from build123d import *

# Parameters (mm, degrees)
SKETCH_2_W      = 48
SKETCH_2_H      = 48
SKETCH_2_W_2    = 40
SKETCH_2_H_2    = 40
EXTRUDE_1_DEPTH = 100
SKETCH_3_W      = 48
SKETCH_3_H      = 48
SKETCH_3_W_2    = 40
SKETCH_3_H_2    = 40
EXTRUDE_2_DEPTH = 40
SKETCH_4_W      = 48
SKETCH_4_H      = 48
SKETCH_4_W_2    = 40
SKETCH_4_H_2    = 40
EXTRUDE_3_DEPTH = 40


with BuildPart() as part:
    # 草图2 → 凸台-拉伸1 (new body)
    with BuildSketch(Plane.XY):
        Rectangle(SKETCH_2_W, SKETCH_2_H)
        Rectangle(SKETCH_2_W_2, SKETCH_2_H_2, mode=Mode.SUBTRACT)
    extrude(amount=EXTRUDE_1_DEPTH)

    # 草图3 → 凸台-拉伸2 (add)
    with BuildSketch(Plane(origin=(24, 0, 0), x_dir=(0, 0, -1), z_dir=(1, 0, 0))):
        with Locations((-50, 0)):
            Rectangle(SKETCH_3_W, SKETCH_3_H)
        with Locations((-50, 0)):
            Rectangle(SKETCH_3_W_2, SKETCH_3_H_2, mode=Mode.SUBTRACT)
    extrude(amount=EXTRUDE_2_DEPTH)

    # 草图4 → 凸台-拉伸3 (add)
    with BuildSketch(Plane(origin=(0, 24, 0), x_dir=(1, 0, 0), z_dir=(0, 1, 0))):
        with Locations((0, -50)):
            Rectangle(SKETCH_4_W, SKETCH_4_H)
        with Locations((0, -50)):
            Rectangle(SKETCH_4_W_2, SKETCH_4_H_2, mode=Mode.SUBTRACT)
    extrude(amount=EXTRUDE_3_DEPTH)


solid = part.part
CAD build for the part. Positions are in the model's coordinates, mm. A direction names the side the tool comes from. Coordinates: 2 decimals unless noted, no trailing zeros. Order: outer loops, then holes, each group sorted by start corner. A loop starts at its lowest first (then second) coordinate and runs counter-clockwise, first axis right, second up. Notation, with made-up numbers: (-32, 9) -> (11, 9) arc R33 ccw to (11, 47) -> close; hole circle Ø11 at (37.5, 88.25). An arc over 180 degrees is marked (long way). Answer in a Markdown table with one row per item.
1) Drill centre lines: line 1 (Z direction, x = 42, y = -14.5); line 2 (Y direction, x = 58, z = 54). Where is each one in solid material? Low to high.
Check values:
| item | result |
|---|---|
| line 1 | 26 to 30, 70 to 74 |
| line 2 | -24 to -20, 20 to 24 |
2) Flat gauge pins, fed straight in: P1, Ø12, axis at x = 12, y = 44, coming from the -Z side; P2, Ø13, axis at y = -7, z = 81, coming from the +X side; P3, Ø20, axis at x = 48.5, y = -8.5, coming from the +Z side. Where does each tip first touch, or does it go through?
Check values:
| item | result |
|---|---|
| P1 | z = 26 |
| P2 | x = 24 |
| P3 | z = 74 |
3) Band-saw the part on A-A (x = 26). List the corners of the cut face in (y, z), and give its area (3 significant figures).
Check values:
| item | result |
|---|---|
| outline | (-24, 26) -> (24, 26) -> (24, 74) -> (-24, 74) -> close; hole (-20, 30) -> (20, 30) -> (20, 70) -> (-20, 70) -> close |
| area | 704 mm2 |
4) Band-saw the part on B-B (y = -10.5). List the corners of the cut face in (x, z).
Check values:
| item | result |
|---|---|
| outline | (-24, 0) -> (-20, 0) -> (-20, 100) -> (-24, 100) -> close; (20, 0) -> (24, 0) -> (24, 26) -> (64, 26) -> (64, 30) -> (24, 30) -> (24, 70) -> (64, 70) -> (64, 74) -> (24, 74) -> (24, 100) -> (20, 100) -> close |
5) Mould opens along Z. For faces 1 (the face through (10, -24, 49)), 2 (the face through (21, 0, 100)), 3 (the face through (44, -20, 50)) say: pulls with the +Z half, pulls with the -Z half, needs draft (parallel to the pull), parting line crosses it, or undercut.
Check values:
| item | result |
|---|---|
| face 1 | needs draft |
| face 2 | pulls with the +Z half |
| face 3 | undercut |
6) Which spindle directions (+Z, -Z, +X, -X, +Y, -Y) get a long thin tool onto all of the face, cutting with end or side? Do faces 4 (the face through (0, 20, 49)), 5 (the face through (24, 0, 87)), 6 (the face through (24, 0, 50)). Say none if no direction does.
Check values:
| item | result |
|---|---|
| face 4 | +Z, -Z |
| face 5 | +Z, +X, +Y, -Y |
| face 6 | +X |
